For this review, take the finished solid that the model builds, in its own axes (mm). Face numbers are marked on the shaded views. A direction names the side the tool comes from. Round coordinates to 2 decimals unless told otherwise and drop trailing zeros. Loops run counter-clockwise (first coordinate to the right, second up) from the corner with the lowest first, then second, coordinate; pieces in that order, holes last. Notation, with made-up numbers: M -23.75,7.25 L 4.25,7.25 A14 ccw 4.25,20.25 Z; hole C 40.25,21.5 d4. An arc over 180 degrees is marked long. One line per question, with ' | ' between items. Start each with the question number.
1) We need section B-B (y = -5). Give the boundary of the cut face in (x, z).
2) We need section D-D (z = 12). Give the boundary of the cut face in (x, y), and give its area (3 significant figures).
3) For pin 1 Ø0.9 at (y, z) = (-4, 17.5) entering from -X; pin 2 Ø5.5 at (y, z) = (-5, -8) entering from +X; pin 3 Ø1 at (x, y) = (-13, -7) entering from +Z, all flat-tipped, find the tip position at first contact; note any pin that passes through.
4) For the marked faces 1, 2 and 3, list the 3-axis set-ups (+Z, -Z, +X, -X, +Y, -Y) from which the entire face can be reached by the end or side of a thin tool; tool diameter is ignored.
5) Mouldability with a two-part tool opening along Z and no side actions: class the marked faces 4, 5 and 6 as pulls with the +Z half, pulls with the -Z half, needs draft (parallel to the pull), parting line crosses it, or undercut.
6) We need section C-C (x = -4.25). Give the boundary of the cut face in (y, z).
7) For probe 1 along Z at (x, y) = (-12.95, -5); probe 2 along Z at (x, y) = (-4.5, -5); probe 3 along X at (y, z) = (-2.5, -9), list the stretches that pass through material, from the lowest coordinate up. Write a range as from..to.
8) We need section A-A (z = -8). Give the boundary of the cut face in (x, y).
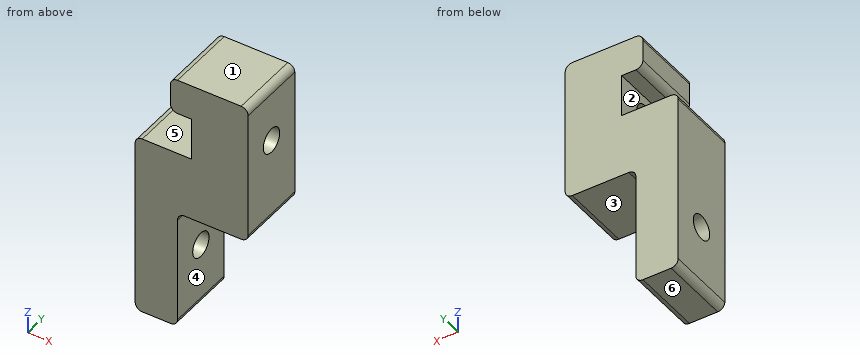
```python
from build123d import *

# Parameters (mm, degrees)
F1_DEPTH = 10
F3_D     = 3.5
F4_R     = 1
F6_D     = 3.5


with BuildPart() as f1:
    # F0 (on Front) → F1 (new body)
    with BuildSketch(Plane.XZ):
        Polygon((-10, 0), (0, 0), (0, 20), (-11, 20), (-11, 15), (-8, 15), (-8, 9), (-16, 9), (-16, -17), (-10, -17), align=None)
    extrude(amount=F1_DEPTH)

    # F3 (through all)
    with Locations(Plane(origin=(-8, 0, 0), x_dir=(0, -1, 0), z_dir=(-1, 0, 0))):
        with Locations((5, 12)):
            Hole(F3_D / 2)

    # F4
    f4_edges = [f1.edges().sort_by_distance(p)[0] for p in [
        (-11, -5, 20),
        (-11, -5, 15),
        (-16, -5, 9),
        (-16, -5, -17),
        (-10, -5, -17),
        (-10, -5, 0),
        (0, -5, 0),
        (0, -5, 20),
    ]]
    fillet(f4_edges, radius=F4_R)

    # F6 (through all)
    with Locations(Plane(origin=(-16, 0, 0), x_dir=(0, -1, 0), z_dir=(-1, 0, 0))):
        with Locations((5, -8)):
            Hole(F6_D / 2)


solid = f1.part
```
Answers below:
1) outline: M -16,-16 A1 ccw -15,-17 L -11,-17 A1 ccw -10,-16 L -10,-9.75 L -16,-9.75 Z; M -16,-6.25 L -10,-6.25 L -10,-1 A1 cw -9,0 L -1,0 A1 ccw 0,1 L 0,10.25 L -8,10.25 L -8,9 L -15,9 A1 ccw -16,8 Z; M -11,16 A1 ccw -10,15 L -8,15 L -8,13.75 L 0,13.75 L 0,19 A1 ccw -1,20 L -10,20 A1 ccw -11,19 Z
2) outline: M -8,-10 L 0,-10 L 0,-6.75 L -8,-6.75 Z; M -8,-3.25 L 0,-3.25 L 0,0 L -8,0 Z | area: 52.0 mm^2
3) pin 1: x = -11 | pin 2: x = -10 | pin 3: z = 9
4) face 1: +Z, +X, -X, +Y, -Y | face 2: -X, +Y, -Y | face 3: -Z, +X, +Y, -Y
5) face 4: needs draft | face 5: undercut | face 6: pulls with the -Z half
6) outline: M -10,0 L 0,0 L 0,20 L -10,20 Z; hole C -5,12 d3.5
7) probe 1: -17..-9.75, -6.25..9 | probe 2: 0..10.25, 13.75..20 | probe 3: -16..-10
8) outline: M -16,-10 L -10,-10 L -10,-6.75 L -16,-6.75 Z; M -16,-3.25 L -10,-3.25 L -10,0 L -16,0 Z
